```python
from build123d import *

# Parameters (mm, degrees)
SKETCH1_R           = 2.5
SKETCH1_R_2         = 1.25
BOSS_EXTRUDE1_DEPTH = 5


with BuildPart() as part:
    # Sketch1 → Boss-Extrude1 (new body)
    # profile 1 of 4: a face of its own
    with BuildSketch(Plane(origin=(0, 0, 0), x_dir=(1, 0, 0), z_dir=(0, 1, 0))):
        Polygon((0, 0), (-70, -80), (-70, 0), align=None)
    # profile 2 of 4: a face of its own
    with BuildSketch(Plane(origin=(0, 0, 0), x_dir=(1, 0, 0), z_dir=(0, 1, 0))):
        Polygon((0, 0), (0, -80), (-70, -80), align=None)
    # profile 3 of 4: a face of its own
    with BuildSketch(Plane(origin=(0, 0, 0), x_dir=(1, 0, 0), z_dir=(0, 1, 0))):
        with BuildLine():
            Line((-32.5, -80), (-37.5, -80))
            Line((-37.5, -80), (-37.5, -88.305370533))
            ThreePointArc((-37.5, -88.305370533), (-35, -85.805370533), (-32.5, -88.305370533))
            Line((-32.5, -88.305370533), (-32.5, -80))
        make_face()
    # profile 4 of 4: a face of its own
    with BuildSketch(Plane(origin=(0, 0, 0), x_dir=(1, 0, 0), z_dir=(0, 1, 0))):
        with Locations((-35, -88.305370533)):
            Circle(SKETCH1_R)
        with Locations(Location((-35, -88.305370533, 0), (0, 0, 270))):
            Circle(SKETCH1_R_2, mode=Mode.SUBTRACT)
    extrude(amount=BOSS_EXTRUDE1_DEPTH)


solid = part.part
```
Could you check a few things on this model? Use its own coordinates, in mm. A direction names the side the tool comes from. Give positions to 0.01 mm unless a question says otherwise; leave off trailing zeros. Order: outer loops, then holes, each group sorted by start corner. A loop starts at its lowest first (then second) coordinate and runs counter-clockwise, first axis right, second up.
Q1. If I drill on line 1 along Z through (x, y) = (-49, 1.1), over which ranges is the centre line in solid material (lowest first)?
Q2. Suppose I cut it at B-B, the plane y = 1.4. Write out the boundary of the cut face in (x, z), and give its area (3 significant figures).
Q3. Suppose I cut it at C-C, the plane x = -50. Write out the boundary of the cut face in (y, z).
Q4. We'd pull the mould along X, two halves only. Please class faces 4 (the flat face through (-35, 2, 0)), 5 (the cylindrical face through (-34.625, 2.465, 89.498)), 6 (the flat face through (-32.5, 2, 84)): +X half, -X half, draft (parallel to the pull), parting line (faces both ways), or undercut.
Q5. Suppose I cut it at A-A, the plane x = -35. Write out the boundary of the cut face in (y, z), and give its area (3 significant figures).
Q6. I'm going to push flat-ended pins straight in: P1, Ø1.5, axis at x = -35, z = 88.31, coming from the -Y side; P2, Ø1.5, axis at y = 1.5, z = 84, coming from the +X side; P3, Ø1.5, axis at x = -17, y = 2.5, coming from the +Z side; P4, Ø2.5, axis at y = 1.5, z = 83.5, coming from the -X side. Where does each tip first touch, or does it pass through?
Q7. For faces 1 (the flat face through (-16, 2, 80)), 2 (the flat face through (-35, 5, 45)), 3 (the flat face through (-54, 2, 80)), which set-ups out of +Z, -Z, +X, -X, +Y, -Y let a thin tool reach every point of the face, with its end or its side?
Solution:
1. line 1: z = 0 to 80
2. outline: (-70, 0) - (0, 0) - (0, 80) - (-32.5, 80) - (-32.5, 88.31) arc R2.5 ccw to (-37.5, 88.31) - (-37.5, 80) - (-70, 80) - close; hole circle Ø2.5 at (-35, 88.31)
2. area: 5,650 mm2
3. outline: (0, 0) - (5, 0) - (5, 80) - (0, 80) - close
4. face 4: draft
4. face 5: undercut
4. face 6: +X half
5. outline: (0, 0) - (5, 0) - (5, 87.06) - (0, 87.06) - close; (0, 89.56) - (5, 89.56) - (5, 90.81) - (0, 90.81) - close
5. area: 442 mm2
6. P1: passes through
6. P2: stops at x = -32.5
6. P3: stops at z = 80
6. P4: stops at x = -37.5
7. face 1: +Z, +X, +Y, -Y
7. face 2: +Z, -Z, +X, -X, +Y
7. face 3: +Z, -X, +Y, -Y
